```python
from build123d import *

# Parameters (mm, degrees)
SKETCH1_W           = 38.1
SKETCH1_H           = 127
BOSS_EXTRUDE1_DEPTH = 6.35
SKETCH2_W           = 6.35
SKETCH2_H           = 12.7
CUT_EXTRUDE1_DEPTH  = 7.35
LPATTERN1_COUNT     = 6
LPATTERN1_PITCH     = 25.4
SKETCH3_W           = 12.7
SKETCH3_H           = 6.35
CUT_EXTRUDE2_DEPTH  = 7.35


with BuildPart() as part:
    # Sketch1 → Boss-Extrude1 (new body)
    with BuildSketch(Plane.XY):
        with Locations((19.05, 63.5)):
            Rectangle(SKETCH1_W, SKETCH1_H)
    extrude(amount=BOSS_EXTRUDE1_DEPTH)

    # Sketch2 → Cut-Extrude1 (cut, through all)
    with BuildSketch(Plane.XY.offset(6.35)):
        with Locations((3.175, 6.35)):
            Rectangle(SKETCH2_W, SKETCH2_H)
        with Locations((34.925, 6.35)):
            Rectangle(SKETCH2_W, SKETCH2_H)
    cut_extrude1 = extrude(amount=-CUT_EXTRUDE1_DEPTH, mode=Mode.SUBTRACT)

    # LPattern1: Cut-Extrude1 ×6
    with Locations(*[(0, i * LPATTERN1_PITCH, 0) for i in range(1, LPATTERN1_COUNT)]):
        add(cut_extrude1, mode=Mode.SUBTRACT)

    # Sketch3 → Cut-Extrude2 (cut, through all)
    with BuildSketch(Plane.XY.offset(6.35)):
        with Locations((12.7, 3.175)):
            Rectangle(SKETCH3_W, SKETCH3_H)
    extrude(amount=-CUT_EXTRUDE2_DEPTH, mode=Mode.SUBTRACT)


solid = part.part
```
Verification items for the finished model (mm, model axes). A direction names the side the tool comes from. Coordinates: 2 decimals unless noted, no trailing zeros. Order: outer loops, then holes, each group sorted by start corner. A loop starts at its lowest first (then second) coordinate and runs counter-clockwise, first axis right, second up. Notation, with made-up numbers: (44.25, 40) -> (63.25, 40) arc R12 cw to (63.25, 59) -> close; hole circle Ø8 at (-22, 86.5). An arc over 180 degrees is marked (long way). Put each result on its own line as item: value. Start each with the question number.
1) Release check for a two-part mould opening along Y. For faces 6 (the flat face through (6.35, 32, 3)), 7 (the flat face through (0, 121, 3)), 8 (the flat face through (3, 114.3, 3)), 9 (the flat face through (19, 127, 3)) record: pulls with the +Y half, pulls with the -Y half, needs draft (parallel to the pull), parting line crosses it, or undercut.
2) Material ranges on L1, parallel to Y at x = 3.5, z = 1; L2, parallel to X at y = 35.5, z = 5.5; L3, parallel to X at y = 6, z = 1.75, recorded low to high.
3) Go/stop test with flat-tipped pins: pin 1 (1.9 mm diameter, centred on y = 29.5, z = 4.5, fed in from -X); pin 2 (1 mm diameter, centred on y = 106, z = 4, fed in from +X); pin 3 (3 mm diameter, centred on x = 15, z = 3.5, fed in from -Y). Record where each tip stops, or that it passes through.
4) Cross-section at A-A (x = 5). Enter the section's corners in (y, z).
5) Cross-section at B-B (y = 61). Enter the section's corners in (x, z), plus the area to 3 significant figures.
6) Tool access check on faces 1 (the flat face through (3, 12.7, 3)), 2 (the flat face through (3, 25.4, 3)), 3 (the flat face through (35, 63.5, 3)), 4 (the flat face through (35, 12.7, 3)), 5 (the flat face through (38.1, 95, 3)). Record the directions out of +Z, -Z, +X, -X, +Y, -Y that give a thin tool (end or side, any length) a straight path to the whole face; none if there is none.
Geometry check:
1. face 6: undercut
1. face 7: needs draft
1. face 8: undercut
1. face 9: pulls with the +Y half
2. L1: y = 12.7 to 25.4, 38.1 to 50.8, 63.5 to 76.2, 88.9 to 101.6, 114.3 to 127
2. L2: x = 6.35 to 31.75
2. L3: x = 19.05 to 31.75
3. pin 1: stops at x = 6.35
3. pin 2: stops at x = 31.75
3. pin 3: stops at y = 6.35
4. outline: (12.7, 0) -> (25.4, 0) -> (25.4, 6.35) -> (12.7, 6.35) -> close; (38.1, 0) -> (50.8, 0) -> (50.8, 6.35) -> (38.1, 6.35) -> close; (63.5, 0) -> (76.2, 0) -> (76.2, 6.35) -> (63.5, 6.35) -> close; (88.9, 0) -> (101.6, 0) -> (101.6, 6.35) -> (88.9, 6.35) -> close; (114.3, 0) -> (127, 0) -> (127, 6.35) -> (114.3, 6.35) -> close
5. outline: (6.35, 0) -> (31.75, 0) -> (31.75, 6.35) -> (6.35, 6.35) -> close
5. area: 161 mm^2
6. face 1: +Z, -Z, -X, -Y
6. face 2: +Z, -Z, -X
6. face 3: +Z, -Z, +X
6. face 4: +Z, -Z, +X, -Y
6. face 5: +Z, -Z, +X, +Y, -Y
